The model under review builds one solid part; all positions refer to its coordinate system, in mm. Round coordinates to 2 decimals unless told otherwise and drop trailing zeros. Loops run counter-clockwise (first coordinate to the right, second up) from the corner with the lowest first, then second, coordinate; pieces in that order, holes last. Notation, with made-up numbers: (5, -10.75) - (44, -10.75) arc R10 cw to (44, 5.25) - close; hole circle Ø7 at (21, 79.25). An arc over 180 degrees is marked (long way). Answer as CSV lines item,"result".
Autodesk Inventor part; units mm, degrees
ref_plane "YZ Plane" through (0, 0, 0) normal (1, 0, 0) x (0, 1, 0)
ref_plane "XZ Plane" through (0, 0, 0) normal (0, 1, 0) x (-1, 0, 0)
ref_plane "XY Plane" through (0, 0, 0) normal (0, 0, 1) x (1, 0, 0)
sketch "Sketch1" plane through (0, 0, 0) normal (0, 0, 1) x (1, 0, 0)
  line L0 (-28.8571, 66) -> (25.1429, 66)
  line L1 (25.1429, 66) -> (25.1429, -114)
  line L2 (25.1429, -114) -> (-28.8571, -114)
  line L3 (-28.8571, -114) -> (-28.8571, 66)
  point P0 (0, 0)
  dimension "d0" = 54
  dimension "d1" = 180
extrude "Extrusion1" add sketch "Sketch1" along normal blind 2
sketch "Sketch2" plane through (0, 0, 2) normal (0, 0, 1) x (1, 0, 0)
  line L0 (25.1429, 66) -> (-28.8571, 66)
  line L1 (-28.8571, 66) -> (-16.8571, 66)
  line L2 (-16.8571, 66) -> (-16.8571, 61)
  line L3 (-16.8571, 61) -> (-28.8571, 61)
  line L4 (-28.8571, 61) -> (-28.8571, 66)
  line L5 (25.1429, 66) -> (13.1429, 66)
  line L6 (13.1429, 66) -> (13.1429, 61)
  line L7 (13.1429, 61) -> (25.1429, 61)
  line L8 (25.1429, 61) -> (25.1429, 66)
  point P0 (0, 0)
  dimension "d4" = 12
  dimension "d5" = 12
  dimension "d6" = 5
extrude "Extrusion2" cut sketch "Sketch2" against normal blind 2
sketch "Sketch3" plane through (0, 0, 2) normal (0, 0, 1) x (1, 0, 0)
  line L0 (-28.8571, 61) -> (-28.8571, -114)
  line L1 (-28.8571, 30) -> (-26.8571, 30)
  line L2 (-26.8571, 30) -> (-26.8571, -6)
  line L3 (-26.8571, -6) -> (-28.8571, -6)
  line L4 (-28.8571, -6) -> (-28.8571, 30)
  line L5 (-28.8571, -42) -> (-26.8571, -42)
  line L6 (-26.8571, -42) -> (-26.8571, -78)
  line L7 (-26.8571, -78) -> (-28.8571, -78)
  line L8 (-28.8571, -78) -> (-28.8571, -42)
  line L9 (25.1429, -114) -> (25.1429, 61)
  line L10 (25.1429, 30) -> (23.1429, 30)
  line L11 (23.1429, 30) -> (23.1429, -6)
  line L12 (23.1429, -6) -> (25.1429, -6)
  line L13 (25.1429, -6) -> (25.1429, 30)
  line L14 (25.1429, -42) -> (23.1429, -42)
  line L15 (23.1429, -42) -> (23.1429, -78)
  line L16 (23.1429, -78) -> (25.1429, -78)
  line L17 (25.1429, -78) -> (25.1429, -42)
  line L18 (-16.8571, 61) -> (-28.8571, 61)
  line L19 (-28.8571, -114) -> (25.1429, -114)
  point P0 (0, 0)
  point P1 (-27.8571, 30)
  point P2 (-27.8571, -42)
  point P3 (-27.8571, -6)
  point P4 (-26.8571, -60)
  point P5 (-27.8571, -78)
  dimension "d10" = 36
  dimension "d11" = 36
  dimension "d12" = 2
  dimension "d13" = 2
  dimension "d14" = 36
  dimension "d15" = 36
extrude "Extrusion3" cut sketch "Sketch3" against normal blind 2
properties part number "front_side"
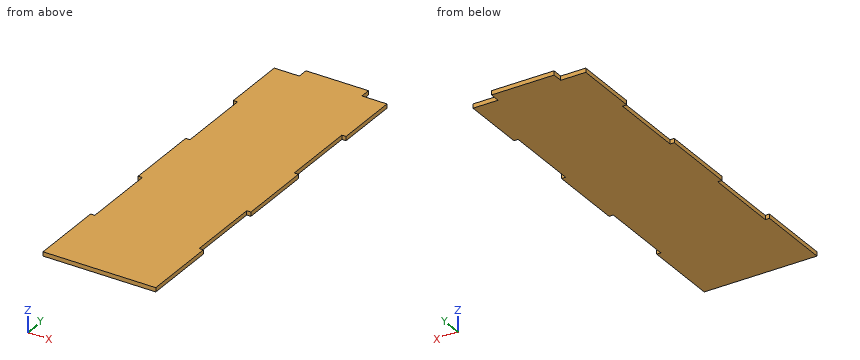
1. Take a section at A-A (z = 1.05). State the section outline as (x, y) points, plus the area to 3 significant figures.
Numbers:
outline,"(-28.86, -114) - (25.14, -114) - (25.14, -78) - (23.14, -78) - (23.14, -42) - (25.14, -42) - (25.14, -6) - (23.14, -6) - (23.14, 30) - (25.14, 30) - (25.14, 61) - (13.14, 61) - (13.14, 66) - (-16.86, 66) - (-16.86, 61) - (-28.86, 61) - (-28.86, 30) - (-26.86, 30) - (-26.86, -6) - (-28.86, -6) - (-28.86, -42) - (-26.86, -42) - (-26.86, -78) - (-28.86, -78) - close"
area,"9,310 mm²"
2. Clearance check with flat-ended pins moving along their axes: pin 1 (0.6 mm diameter, centred on y = 63.5, z = 0.5, fed in from -X); pin 2 (1 mm diameter, centred on y = 16, z = 1, fed in from -X); pin 3 (1 mm diameter, centred on x = -22, z = 1, fed in from +Y). State where each tip first meets the part, or that it passes through.
Numbers:
pin 1,"stops at x = -16.86"
pin 2,"stops at x = -26.86"
pin 3,"stops at y = 61"
3. Take a section at B-B (y = 13). State the section outline as (x, z) points.
Numbers:
outline,"(-26.86, 0) - (23.14, 0) - (23.14, 2) - (-26.86, 2) - close"
4. Take a section at C-C (x = 20.5). State the section outline as (y, z) points, plus the area to 3 significant figures.
Numbers:
outline,"(-114, 0) - (61, 0) - (61, 2) - (-114, 2) - close"
area,"350 mm²"
5. Wall thickness on probe 1 along X at (y, z) = (-70.5, 1.55); probe 2 along Y at (x, z) = (15.5, 1.35): over which ranges is each line inside the solid? List them lowest first.
Numbers:
probe 1,"x = -26.86 to 23.14"
probe 2,"y = -114 to 61"
